Design review of the part built by this model. Coordinates are the model's own, in mm. Coordinates: 2 decimals unless noted, no trailing zeros. Loops run counter-clockwise (first coordinate to the right, second up) from the corner with the lowest first, then second, coordinate; pieces in that order, holes last. Notation, with made-up numbers: (38.25, 82.25) - (42.25, 82.25) arc R23 ccw to (42.25, 103.25) - close; hole circle Ø3 at (81, 9). An arc over 180 degrees is marked (long way). One line per question, with ' | ' between items.
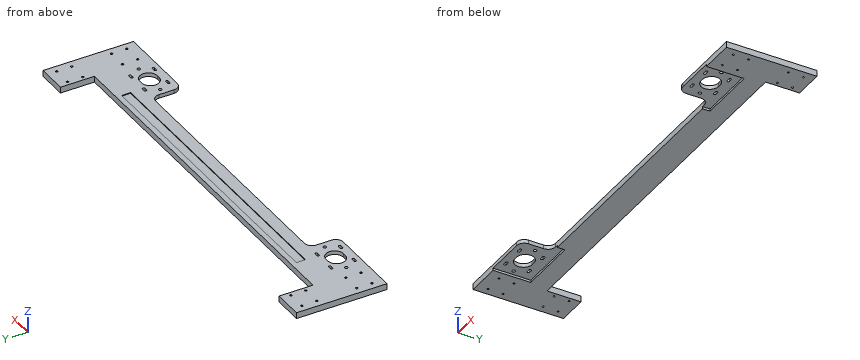
from build123d import *

# Parameters (mm, degrees)
BOSS_EXTRUDE1_DEPTH         = 8
SKETCH5_W                   = 120
SKETCH5_H                   = 40
BOSS_EXTRUDE4_DEPTH         = 8
M3_TAPPED_HOLE2_D           = 2.5
M3_TAPPED_HOLE2_CSINK_D     = 3.05
M3_TAPPED_HOLE2_CSINK_ANGLE = 90
SKETCH24_W                  = 400
SKETCH24_H                  = 12
CUT_EXTRUDE4_DEPTH          = 1
M5_TAPPED_HOLE3_D           = 4.2
M5_TAPPED_HOLE3_CSINK_D     = 5.05
M5_TAPPED_HOLE3_CSINK_ANGLE = 90
MIRROR3_COPY_1_D            = 2.5
MIRROR3_COPY_1_CSINK_D      = 3.05
MIRROR3_COPY_1_CSINK_ANGLE  = 90
MIRROR3_COPY_2_D            = 2.5
MIRROR3_COPY_2_CSINK_D      = 3.05
MIRROR3_COPY_2_CSINK_ANGLE  = 90
SKETCH27_W                  = 54.08
SKETCH27_H                  = 3
CUT_EXTRUDE6_DEPTH          = 50


with BuildPart() as part:
    # Sketch1 → Boss-Extrude1 (new body)
    with BuildSketch(Plane.XY):
        with BuildLine():
            Line((-250, -33.879809267), (-240, -33.879809267))
            Line((-240, -33.879809267), (-200, -33.879809267))
            Line((-200, -33.879809267), (-190, -33.879809267))
            ThreePointArc((-190, -33.879809267), (-182.928932188, -30.950877079), (-180, -23.879809267))
            Line((-180, -23.879809267), (-180, -3.879809267))
            ThreePointArc((-180, -3.879809267), (-177.071067812, 3.191258545), (-170, 6.120190733))
            Line((-170, 6.120190733), (-150, 6.120190733))
            Line((-150, 6.120190733), (150, 6.120190733))
            Line((150, 6.120190733), (170, 6.120190733))
            ThreePointArc((170, 6.120190733), (177.071067812, 3.191258545), (180, -3.879809267))
            Line((180, -3.879809267), (180, -23.879809267))
            ThreePointArc((180, -23.879809267), (182.928932188, -30.950877079), (190, -33.879809267))
            Line((190, -33.879809267), (200, -33.879809267))
            Line((200, -33.879809267), (240, -33.879809267))
            Line((240, -33.879809267), (250, -33.879809267))
            Line((250, -33.879809267), (250, 36.120190733))
            Line((250, 36.120190733), (250, 41.120190733))
            Line((250, 41.120190733), (-250, 41.120190733))
            Line((-250, 41.120190733), (-250, 36.120190733))
            Line((-250, 36.120190733), (-250, -23.879809267))
            Line((-250, -23.879809267), (-250, -33.879809267))
        make_face()
        with BuildLine():
            ThreePointArc((-230.5, -27.479809267), (-232.1, -25.879809267), (-230.5, -24.279809267))
            Line((-230.5, -24.279809267), (-226.5, -24.279809267))
            ThreePointArc((-226.5, -24.279809267), (-224.9, -25.879809267), (-226.5, -27.479809267))
            Line((-226.5, -27.479809267), (-230.5, -27.479809267))
        make_face(mode=Mode.SUBTRACT)
        with BuildLine():
            ThreePointArc((-195.5, -24.279809267), (-193.9, -25.879809267), (-195.5, -27.479809267))
            Line((-195.5, -27.479809267), (-199.5, -27.479809267))
            ThreePointArc((-199.5, -27.479809267), (-201.1, -25.879809267), (-199.5, -24.279809267))
            Line((-199.5, -24.279809267), (-195.5, -24.279809267))
        make_face(mode=Mode.SUBTRACT)
        with BuildLine():
            Line((-215, 1.220190733), (-211, 1.220190733))
            ThreePointArc((-211, 1.220190733), (-199.4, -10.379809267), (-211, -21.979809267))
            Line((-211, -21.979809267), (-215, -21.979809267))
            ThreePointArc((-215, -21.979809267), (-226.6, -10.379809267), (-215, 1.220190733))
        make_face(mode=Mode.SUBTRACT)
        with BuildLine():
            ThreePointArc((195.5, -27.479809267), (193.9, -25.879809267), (195.5, -24.279809267))
            Line((195.5, -24.279809267), (199.5, -24.279809267))
            ThreePointArc((199.5, -24.279809267), (201.1, -25.879809267), (199.5, -27.479809267))
            Line((199.5, -27.479809267), (195.5, -27.479809267))
        make_face(mode=Mode.SUBTRACT)
        with BuildLine():
            ThreePointArc((230.5, -24.279809267), (232.1, -25.879809267), (230.5, -27.479809267))
            Line((230.5, -27.479809267), (226.5, -27.479809267))
            ThreePointArc((226.5, -27.479809267), (224.9, -25.879809267), (226.5, -24.279809267))
            Line((226.5, -24.279809267), (230.5, -24.279809267))
        make_face(mode=Mode.SUBTRACT)
        with BuildLine():
            Line((215, -21.979809267), (211, -21.979809267))
            ThreePointArc((211, -21.979809267), (199.4, -10.379809267), (211, 1.220190733))
            Line((211, 1.220190733), (215, 1.220190733))
            ThreePointArc((215, 1.220190733), (226.6, -10.379809267), (215, -21.979809267))
        make_face(mode=Mode.SUBTRACT)
        with BuildLine():
            Line((-226.5, 3.520190733), (-230.5, 3.520190733))
            ThreePointArc((-230.5, 3.520190733), (-232.1, 5.120190733), (-230.5, 6.720190733))
            Line((-230.5, 6.720190733), (-226.5, 6.720190733))
            ThreePointArc((-226.5, 6.720190733), (-224.9, 5.120190733), (-226.5, 3.520190733))
        make_face(mode=Mode.SUBTRACT)
        with BuildLine():
            Line((-199.5, 6.720190733), (-195.5, 6.720190733))
            ThreePointArc((-195.5, 6.720190733), (-193.9, 5.120190733), (-195.5, 3.520190733))
            Line((-195.5, 3.520190733), (-199.5, 3.520190733))
            ThreePointArc((-199.5, 3.520190733), (-201.1, 5.120190733), (-199.5, 6.720190733))
        make_face(mode=Mode.SUBTRACT)
        with BuildLine():
            Line((199.5, 3.520190733), (195.5, 3.520190733))
            ThreePointArc((195.5, 3.520190733), (193.9, 5.120190733), (195.5, 6.720190733))
            Line((195.5, 6.720190733), (199.5, 6.720190733))
            ThreePointArc((199.5, 6.720190733), (201.1, 5.120190733), (199.5, 3.520190733))
        make_face(mode=Mode.SUBTRACT)
        with BuildLine():
            Line((226.5, 6.720190733), (230.5, 6.720190733))
            ThreePointArc((230.5, 6.720190733), (232.1, 5.120190733), (230.5, 3.520190733))
            Line((230.5, 3.520190733), (226.5, 3.520190733))
            ThreePointArc((226.5, 3.520190733), (224.9, 5.120190733), (226.5, 6.720190733))
        make_face(mode=Mode.SUBTRACT)
    extrude(amount=BOSS_EXTRUDE1_DEPTH)

    # Sketch5 → Boss-Extrude4 (add)
    with BuildSketch(Plane(origin=(-195.879809267, 36.120190733, 8), x_dir=(0, -1, 0), z_dir=(0, 0, -1))):
        with Locations((10, 74.120190733)):
            Rectangle(SKETCH5_W, SKETCH5_H)
    boss_extrude4 = extrude(amount=BOSS_EXTRUDE4_DEPTH)

    # M3 Tapped Hole2 (through all)
    with Locations(Plane(origin=(-280.5, 53.620190733, 8), x_dir=(1, 0, 0), z_dir=(0, 0, 1))):
        with Locations((0, 0), (25, 20), (25, 0), (0, 20)):
            m3_tapped_hole2 = CounterSinkHole(M3_TAPPED_HOLE2_D / 2, M3_TAPPED_HOLE2_CSINK_D / 2, counter_sink_angle=M3_TAPPED_HOLE2_CSINK_ANGLE)

    # Mirror1: Boss-Extrude4, M3 Tapped Hole2 across plane
    add(boss_extrude4.mirror(Plane(origin=(0, 0, 0), x_dir=(0, 0, 1), z_dir=(1, 0, 0))))
    add(m3_tapped_hole2.mirror(Plane(origin=(0, 0, 0), x_dir=(0, 0, 1), z_dir=(1, 0, 0))), mode=Mode.SUBTRACT)

    # Sketch24 → Cut-Extrude4 (cut)
    with BuildSketch(Plane.XY.offset(8)):
        with Locations((0, 28.120190733)):
            Rectangle(SKETCH24_W, SKETCH24_H)
    extrude(amount=-CUT_EXTRUDE4_DEPTH, mode=Mode.SUBTRACT)

    # M5 Tapped Hole3 (through all)
    with Locations(Plane(origin=(0, 0, 0), x_dir=(-1, 0, 0), z_dir=(0, 0, -1))):
        with Locations((237.58, -10.379809267), (188.42, -10.379809267), (-188.42, -10.379809267), (-237.58, -10.379809267)):
            CounterSinkHole(M5_TAPPED_HOLE3_D / 2, M5_TAPPED_HOLE3_CSINK_D / 2, counter_sink_angle=M5_TAPPED_HOLE3_CSINK_ANGLE)

    # Mirror2: M3 Tapped Hole2 across plane
    add(m3_tapped_hole2.mirror(Plane(origin=(0, 27.120190733, 0), x_dir=(0, 0, 1), z_dir=(0, -1, 0))), mode=Mode.SUBTRACT)

    # Mirror3 copy 1 (through all)
    with Locations(Plane(origin=(280.5, 0.620190733, 8), x_dir=(-1, 0, 0), z_dir=(0, 0, 1))):
        with Locations((0, 0), (25, 20), (25, 0), (0, 20)):
            CounterSinkHole(MIRROR3_COPY_1_D / 2, MIRROR3_COPY_1_CSINK_D / 2, counter_sink_angle=MIRROR3_COPY_1_CSINK_ANGLE)

    # Mirror3 copy 2 (through all)
    with Locations(Plane(origin=(280.5, 53.620190733, 8), x_dir=(-1, 0, 0), z_dir=(0, 0, 1))):
        with Locations((0, 0), (25, -20), (25, 0), (0, -20)):
            CounterSinkHole(MIRROR3_COPY_2_D / 2, MIRROR3_COPY_2_CSINK_D / 2, counter_sink_angle=MIRROR3_COPY_2_CSINK_ANGLE)

    # Sketch27 → Cut-Extrude6 (cut)
    with BuildSketch(Plane.XZ.offset(33.879809267)):
        with Locations((217.04, 1.5)):
            Rectangle(SKETCH27_W, SKETCH27_H)
        Polygon((166, -7.690904526), (244.08, -7.690904526), (244.08, 0), (190, 0), (190, 3), (166, 3), align=None)
    cut_extrude6 = extrude(amount=-CUT_EXTRUDE6_DEPTH, mode=Mode.SUBTRACT)

    # Mirror4: Cut-Extrude6 across plane
    add(cut_extrude6.mirror(Plane(origin=(0, 0, 0), x_dir=(0, 0, 1), z_dir=(1, 0, 0))), mode=Mode.SUBTRACT)


solid = part.part
Q1. Take a section at A-A (x = -79). Give the boundary of the cut face in (y, z), plus the area to 3 significant figures.
Returned:
outline: (6.12, 0) - (41.12, 0) - (41.12, 8) - (34.12, 8) - (34.12, 7) - (22.12, 7) - (22.12, 8) - (6.12, 8) - close | area: 268 mm²
Q2. To check wall thickness, follow line 1 along Y through (x, z) = (-230.5, 7); line 2 along X through (y, z) = (-14.5, 4.5); line 3 along X through (y, z) = (-26.5, 2.25). State the ranges of each line that lie inside material, in increasing order.
Returned:
line 1: y = -33.88 to -27.48, -24.28 to 3.52, 6.72 to 41.12 | line 2: x = -290 to -225.84, -200.16 to -180, 180 to 200.16, 225.84 to 290 | line 3: x = -290 to -244.08, 244.08 to 290
Q3. For pin 1 (2.5 mm diameter, centred on x = 71.5, z = 3, fed in from -Y); pin 2 (1.2 mm diameter, centred on x = 198.5, z = 6.5, fed in from +Y); pin 3 (6 mm diameter, centred on x = 8, y = 28.5, fed in from +Z), all flat-tipped, find the tip position at first contact; note any pin that passes through.
Returned:
pin 1: stops at y = 6.12 | pin 2: stops at y = 41.12 | pin 3: stops at z = 7
